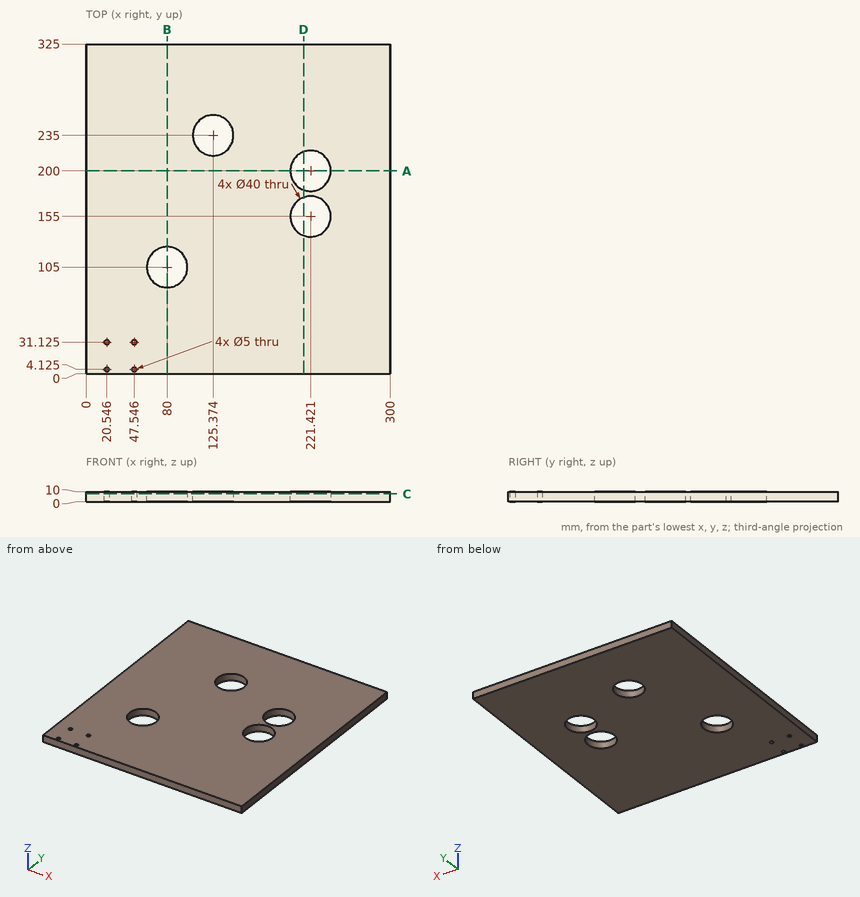
Can you work these out from the drawing? Everything is in mm from the part's minimum corner. Give positions to 0.01 mm unless a question says otherwise; leave off trailing zeros. Order: outer loops, then holes, each group sorted by start corner. A loop starts at its lowest first (then second) coordinate and runs counter-clockwise, first axis right, second up. Notation, with made-up numbers: M 73.5,68 L 114.5,68 A17 ccw 114.5,82 Z; hole C 18,36 d10. An arc over 180 degrees is marked long. One line per question, with ' | ' between items.
1. I want a section at A-A (y = 200). List the corners of the cut face in (x, z) for me.
Results:
outline: M 0,0 L 201.42,0 L 201.42,10 L 0,10 Z; M 241.42,0 L 300,0 L 300,10 L 241.42,10 Z
2. If I drill on line 1 (Y direction, x = 239, z = 8.25) (1 decimal); line 2 (X direction, y = 168.5, z = 0.5) (1 decimal); line 3 (X direction, y = 104, z = 6) (1 decimal), over which ranges is the centre line in solid material (lowest first)?
Results:
line 1: 0 to 145.5, 164.5 to 190.5, 209.5 to 325 | line 2: 0 to 206.7, 236.2 to 300 | line 3: 0 to 60, 100 to 300
3. I want a section at D-D (x = 214.5). List the corners of the cut face in (y, z) for me (1 decimal).
Results:
outline: M 0,0 L 136.2,0 L 136.2,10 L 0,10 Z; M 173.8,0 L 181.2,0 L 181.2,10 L 173.8,10 Z; M 218.8,0 L 325,0 L 325,10 L 218.8,10 Z
4. I want a section at B-B (x = 80). List the corners of the cut face in (y, z) for me.
Results:
outline: M 0,0 L 85,0 L 85,10 L 0,10 Z; M 125,0 L 325,0 L 325,10 L 125,10 Z
5. I want a section at C-C (z = 7.75). Give the number of separate pieces and of enclosed holes in the cut face, and give its area (3 significant figures).
Results:
separate pieces: 1 | enclosed holes: 8 | area: 92,400 mm²
